from build123d import *

# Parameters (mm, degrees)
F0_W     = 100
F0_H     = 100
F1_DEPTH = 70
F2_W     = 98
F2_H     = 98
F3_DEPTH = 69
F4_W     = 31.666
F4_H     = 1
F4_W_2   = 1
F4_W_3   = 32.668
F4_H_2   = 32.668
F4_H_3   = 31.666
F5_DEPTH = 69
F7_DEPTH = 100.001
F8_ANGLE = 180


with BuildPart() as f1:
    # F0 (on Top) → F1 (new body)
    with BuildSketch(Plane.XY):
        Rectangle(F0_W, F0_H)
    extrude(amount=F1_DEPTH)

    # F2 (on face) → F3 (cut)
    with BuildSketch(Plane.XY.offset(70)):
        Rectangle(F2_W, F2_H)
    extrude(amount=-F3_DEPTH, mode=Mode.SUBTRACT)

    # F4 (on face) → F5 (join)
    with BuildSketch(Plane.XY.offset(1)):
        with Locations((33.167, -16.834)):
            Rectangle(F4_W, F4_H)
        with Locations((16.834, -16.834)):
            Rectangle(F4_W_2, F4_H)
        with Locations((0, -16.834)):
            Rectangle(F4_W_3, F4_H)
        with Locations((-16.834, -16.834)):
            Rectangle(F4_W_2, F4_H)
        with Locations((-33.167, -16.834)):
            Rectangle(F4_W, F4_H)
        with Locations((-16.834, 0)):
            Rectangle(F4_W_2, F4_H_2)
        with Locations((16.834, 0)):
            Rectangle(F4_W_2, F4_H_2)
        with Locations((33.167, 16.834)):
            Rectangle(F4_W, F4_H)
        with Locations((16.834, 16.834)):
            Rectangle(F4_W_2, F4_H)
        with Locations((0, 16.834)):
            Rectangle(F4_W_3, F4_H)
        with Locations((-16.834, 16.834)):
            Rectangle(F4_W_2, F4_H)
        with Locations((-33.167, 16.834)):
            Rectangle(F4_W, F4_H)
        with Locations((-16.834, 33.167)):
            Rectangle(F4_W_2, F4_H_3)
        with Locations((16.834, 33.167)):
            Rectangle(F4_W_2, F4_H_3)
    extrude(amount=F5_DEPTH)

    # F6 (on face) → F7 (cut, through all)
    with BuildSketch(Plane(origin=(-50, 0, 0), x_dir=(0, -1, 0), z_dir=(-1, 0, 0))):
        Polygon((-50, 18.0460233241), (15.8534999937, 70), (-50, 70), align=None)
    extrude(amount=-F7_DEPTH, mode=Mode.SUBTRACT)


with BuildPart() as f1_1:
    # F8: moved
    add(f1.part.rotate(Axis((16.334, 16.334, 35.5), (0, 0, -1)), F8_ANGLE))


solid = f1_1.part
Here's how the part is built. I have some questions about the finished solid (model axes, mm). A direction names the side the tool comes from. Round coordinates to 2 decimals unless told otherwise and drop trailing zeros. Order: outer loops, then holes, each group sorted by start corner. A loop starts at its lowest first (then second) coordinate and runs counter-clockwise, first axis right, second up. Notation, with made-up numbers: M -15,-13 L 12,-13 A34 ccw 12,25 Z; hole C -28.75,-7 d1. An arc over 180 degrees is marked long. Return JSON: item names as keys, results as strings. Group by question number.
1. On a 3-axis mill with a long thin cutter (end or side, diameter ignored), from which of +Z, -Z, +X, -X, +Y, -Y can I reach the whole of each face in a straight line? I mean faces 5 (the face through (33, -17.332, 9)), 6 (the face through (50.002, 3, 17)). Say none if no direction works.
2. If we section it at A-A on z = 16: State how many separate pieces and enclosed holes the cut face has, then the cut area to 3 significant figures.
3. Please list where these lines run through material, in increasing order: probe 1 along Y at (x, z) = (70, 25); probe 2 along X at (y, z) = (41, 8.5).
4. If we section it at C-C on x = 10: List the corners of the cut face in (y, z) for me, then the cut area to 3 significant figures.
5. If we mould it in two halves opening along X, with no side actions, what happens to faces 1 (the face through (-17.332, 44, 27)), 2 (the face through (66, 16.334, 22)), 3 (the face through (33, 82, 70)), 4 (the face through (-1, 49.002, 35))? For each: pulls with the +X half, pulls with the -X half, needs draft (parallel to the pull), parting line crosses it, or undercut.
6. If we section it at D-D on z = 62.5: List the corners of the cut face in (x, y) for me, then the cut area to 3 significant figures.
7. If we section it at B-B on y = 61.5: List the corners of the cut face in (x, z) for me.
8. I'm going to push flat-ended pins straight in: pin 1 Ø9.5 at (x, y) = (-7.5, 1) entering from +Z; pin 2 Ø9.5 at (x, z) = (65, 28.5) entering from -Y; pin 3 Ø6 at (x, z) = (17, 37.5) entering from -Y. Where does each tip first touch, or does it pass through?
Reply:
{
 "1": {"face 5": "+Z, -Z, +X, -X, -Y", "face 6": "+Z"},
 "2": {"separate pieces": "1", "enclosed holes": "7", "area": "721 mm^2"},
 "3": {"probe 1": "15.33 to 16.33, 49 to 50, 81.67 to 82.67", "probe 2": "-17.33 to -16.33, 15.33 to 16.33, 49 to 50, 81.67 to 82.67"},
 "4": {"outline": "M -17.33,0 L 82.67,0 L 82.67,70 L 81.67,70 L 81.67,1 L 50,1 L 50,70 L 49,70 L 49,1 L 16.33,1 L 16.33,44.61 L 15.33,43.82 L 15.33,1 L -16.33,1 L -16.33,18.83 L -17.33,18.05 Z", "area": "299 mm^2"},
 "5": {"face 1": "pulls with the -X half", "face 2": "undercut", "face 3": "needs draft", "face 4": "undercut"},
 "6": {"outline": "M -17.33,39.01 L -16.33,39.01 L -16.33,49 L 15.33,49 L 15.33,39.01 L 16.33,39.01 L 16.33,49 L 49,49 L 49,39.01 L 50,39.01 L 50,49 L 81.67,49 L 81.67,39.01 L 82.67,39.01 L 82.67,82.67 L -17.33,82.67 Z; hole M -16.33,50 L 81.67,50 L 81.67,81.67 L -16.33,81.67 Z", "area": "303 mm^2"},
 "7": {"outline": "M -17.33,0 L 82.67,0 L 82.67,70 L 81.67,70 L 81.67,1 L -16.33,1 L -16.33,70 L -17.33,70 Z"},
 "8": {"pin 1": "z = 1", "pin 2": "y = 15.33", "pin 3": "y = 3.62"}
}
